Source: CAD feature listing. Evaluate the final solid. Frame: model axes, mm. Face numbers are marked on the shaded views. A direction names the side the tool comes from. Give positions to 0.01 mm unless a question says otherwise; leave off trailing zeros. Order: outer loops, then holes, each group sorted by start corner. A loop starts at its lowest first (then second) coordinate and runs counter-clockwise, first axis right, second up. Notation, with made-up numbers: M 31,21.5 L 56,21.5 A19 ccw 56,52.5 Z; hole C 79.5,32 d11. An arc over 180 degrees is marked long. Answer in a Markdown table with one row per item. Add a question column.
(1) Section query A-A, the plane z = 50. Return loops of the section in (x, y), plus the area to 3 significant figures.
(2) Section query C-C, the plane z = 253. Return loops of the section in (x, y).
(3) Section query B-B, the plane x = 93.5. Return loops of the section in (y, z), plus the area to 3 significant figures.
(4) Set-up query: the marked faces 1 and 2. Return all of +Z, -Z, +X, -X, +Y, -Y with unobstructed straight access to the full face (end or side cutting, diameter ignored); none if empty.
(5) Pin query (flat end, axial travel): P1, Ø6, axis at x = 50.5, z = 243.5, coming from the -Y side; P2, Ø7, axis at x = 118.5, y = -273, coming from the +Z side. Return the tip coordinate at first contact, or that it passes through.
(6) Material intervals for line 1 along Y through (x, z) = (74, 380.5); line 2 along X through (y, z) = (-247, 243.5), sorted ascending.
(7) Section query D-D, the plane y = -246. Return loops of the section in (x, z), plus the area to 3 significant figures.
from build123d import *

# Parameters (mm, degrees)
F0_W     = 260
F0_H     = 420
F1_DEPTH = 230
F3_DEPTH = 420
F4_W     = 160
F4_H     = 76.108451
F5_DEPTH = 360


with BuildPart() as f1:
    # F0 (on Front) → F1 (new body)
    with BuildSketch(Plane.XZ):
        with Locations((130, 210)):
            Rectangle(F0_W, F0_H)
    extrude(amount=F1_DEPTH)

    # F2 (on Top) → F3 (join, through all)
    with BuildSketch(Plane.XY):
        with BuildLine():
            Line((260, -230), (0, -230))
            Line((0, -230), (0, -236))
            Line((0, -236), (24.574561, -253.207293))
            ThreePointArc((24.574561, -253.207293), (130, -278), (235.425439, -253.207293))
            Line((235.425439, -253.207293), (260, -236))
            Line((260, -236), (260, -230))
        make_face()
    extrude(amount=F3_DEPTH)

    # F4 (on face) → F5 (cut)
    with BuildSketch(Plane.XY.offset(420)):
        with Locations((130, -302.115488)):
            Rectangle(F4_W, F4_H)
    extrude(amount=-F5_DEPTH, mode=Mode.SUBTRACT)


solid = f1.part
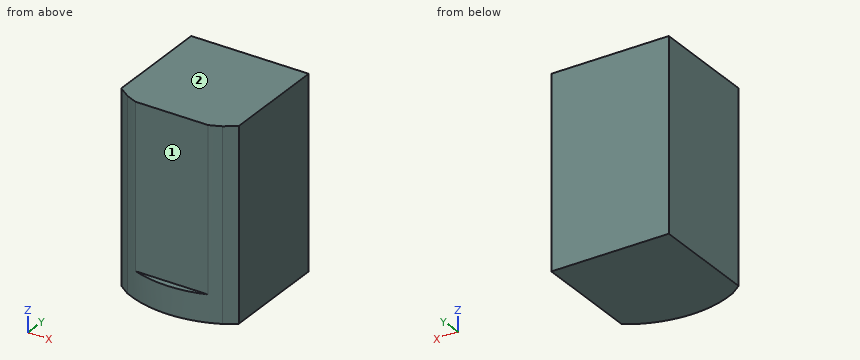
Values follow:
| question | item | result |
|---|---|---|
| 1 | outline | M 0,-236 L 24.57,-253.21 A236.55 ccw 235.43,-253.21 L 260,-236 L 260,0 L 0,0 Z |
| 1 | area | 68,900 mm² |
| 2 | outline | M 0,-236 L 24.57,-253.21 A236.55 ccw 50,-264.06 L 210,-264.06 A236.55 ccw 235.43,-253.21 L 260,-236 L 260,0 L 0,0 Z |
| 3 | outline | M -275.17,0 L 0,0 L 0,420 L -264.06,420 L -264.06,60 L -275.17,60 Z |
| 3 | area | 112,000 mm² |
| 4 | face 1 | +Z, +X, -X, -Y |
| 4 | face 2 | +Z, +X, -X, +Y, -Y |
| 5 | P1 | stops at y = -264.06 |
| 5 | P2 | stops at z = 60 |
| 6 | line 1 | y = -264.06 to 0 |
| 6 | line 2 | x = 15.71 to 244.29 |
| 7 | outline | M 14.28,0 L 245.72,0 L 245.72,420 L 14.28,420 Z |
| 7 | area | 97,200 mm² |
